```python
from build123d import *

# Parameters (mm, degrees)
BASPROSKE_W         = 12
BASPROSKE_H         = 14
TOOTHCUT_DEPTH      = 24.151673806
TEETHCUTS_COUNT     = 12
TEETHCUTS_ANGLE     = 330
BORSKE_R            = 2.5
BORE_DEPTH          = 50.0000508
CUT_EXTRUDE_1_DEPTH = 5


with BuildPart() as part:
    # BasProSke → Base-Revolve (revolve)
    with BuildSketch(Plane(origin=(0, 0, 0), x_dir=(1, 0, 0), z_dir=(0, 1, 0)), mode=Mode.PRIVATE) as base_revolve_sk:
        with Locations((6, 7)):
            Rectangle(BASPROSKE_W, BASPROSKE_H)
    revolve(base_revolve_sk.sketch.rotate(Axis((-10, 0, 0), (1, 0, 0)), 180), axis=Axis((-10, 0, 0), (1, 0, 0)))

    # TooCutSke → ToothCut (cut, through all)
    with BuildSketch(Plane(origin=(0, 0, 0), x_dir=(0, 0, -1), z_dir=(1, 0, 0))):
        with BuildLine():
            ThreePointArc((1.111908866, 9.433698091), (0, 9.499), (-1.111908866, 9.433698091))
            ThreePointArc((-1.111908866, 9.433698091), (-1.651516138, 11.821129337), (-3.298149691, 13.632096456))
            ThreePointArc((-3.298149691, 13.632096456), (0, 14.0254), (3.298149691, 13.632096456))
            ThreePointArc((3.298149691, 13.632096456), (1.651516138, 11.821129337), (1.111908866, 9.433698091))
        make_face()
    toothcut = extrude(amount=TOOTHCUT_DEPTH, mode=Mode.SUBTRACT)

    # TeethCuts: ToothCut ×12 about axis
    teethcuts_axis = Axis((-10, 0, 0), (1, 0, 0))
    for i in range(1, TEETHCUTS_COUNT):
        add(toothcut.rotate(teethcuts_axis, i * TEETHCUTS_ANGLE / (TEETHCUTS_COUNT - 1)), mode=Mode.SUBTRACT)

    # BorSke → Bore (cut, symmetric)
    with BuildSketch(Plane(origin=(0, 0, 0), x_dir=(0, 0, -1), z_dir=(1, 0, 0))):
        with Locations(Location((0, 0, 0), (0, 0, 180))):
            Circle(BORSKE_R)
    extrude(amount=BORE_DEPTH, both=True, mode=Mode.SUBTRACT)

    # Эскиз1 → Вырез-Вытянуть1 (cut)
    with BuildSketch(Plane(origin=(12, 0, 0), x_dir=(0, 0, -1), z_dir=(1, 0, 0))):
        Polygon((8.948929172, 0), (4.474464586, 7.75), (-4.474464586, 7.75), (-8.948929172, 0), (-4.474464586, -7.75), (4.474464586, -7.75), align=None)
    extrude(amount=-CUT_EXTRUDE_1_DEPTH, mode=Mode.SUBTRACT)


solid = part.part
```
Can you work these out from the model? Positions are in its coordinate system, mm. A direction names the side the tool comes from. Coordinates: 2 decimals unless noted, no trailing zeros. Loops run counter-clockwise (first coordinate to the right, second up) from the corner with the lowest first, then second, coordinate; pieces in that order, holes last. Notation, with made-up numbers: (61.25, -31.5) -> (93.25, -31.5) arc R20 cw to (93.25, -27.5) -> close; hole circle Ø8 at (29, -35.75). An arc over 180 degrees is marked (long way). Put each result on its own line as item: value. Start each with the question number.
Q1. I'm going to push flat-ended pins straight in: P1, Ø5.5, axis at x = 9, z = -2, coming from the +Y side; P2, Ø5.5, axis at x = 8.5, z = 1, coming from the -Y side; P3, Ø2, axis at x = 9, z = 8, coming from the +Y side; P4, Ø1, axis at y = -7.5, z = -5, coming from the -X side. Where does each tip first touch, or does it pass through?
Q2. For faces 1 (the face through (3.5, -0.1, -2.5)), 2 (the face through (9.535, 3.821, -6.743)), which set-ups out of +Z, -Z, +X, -X, +Y, -Y let a thin tool reach every point of the face, with its end or its side?
Q3. I want a section at A-A (z = 0). Write out the boundary of the cut face in (x, y), plus the area to 3 significant figures.
Q4. I want a section at C-C (z = -11.25). Write out the boundary of the cut face in (x, y), plus the area to 3 significant figures.
Q5. I want a section at B-B (y = -0.5). Write out the boundary of the cut face in (x, z).
Q6. If I drill on line 1 (Y direction, x = 2.25, z = 8.25); line 2 (Y direction, x = 2.25, z = 8); line 3 (Z direction, x = 8.5, y = -3.5), over which ranges is the centre line in solid material (lowest first)? Write a range as [from, to].
Taken from the geometry:
1. P1: stops at y = 13.61
1. P2: stops at y = -13.61
1. P3: stops at y = 10.07
1. P4: stops at x = 0
2. face 1: +X, -X
2. face 2: +X
3. outline: (0, -9.5) -> (12, -9.5) -> (12, -7.75) -> (7, -7.75) -> (7, -2.5) -> (0, -2.5) -> close; (0, 2.5) -> (7, 2.5) -> (7, 7.75) -> (12, 7.75) -> (12, 9.5) -> (0, 9.5) -> close
3. area: 115 mm2
4. outline: (0, -4.48) -> (12, -4.48) -> (12, -1.4) -> (0, -1.4) -> close; (0, 1.4) -> (12, 1.4) -> (12, 4.48) -> (0, 4.48) -> close
4. area: 74.0 mm2
5. outline: (0, -9.49) -> (12, -9.49) -> (12, -8.66) -> (7, -8.66) -> (7, -2.45) -> (0, -2.45) -> close; (0, 2.45) -> (7, 2.45) -> (7, 8.66) -> (12, 8.66) -> (12, 9.49) -> (0, 9.49) -> close
6. line 1: y = [-9.86, -6.08], [-4.71, 4.71], [6.08, 9.86]
6. line 2: y = [-9.76, -5.91], [-5.12, 5.12], [5.91, 9.76]
6. line 3: z = [-13.56, -6.93], [6.93, 13.56]
